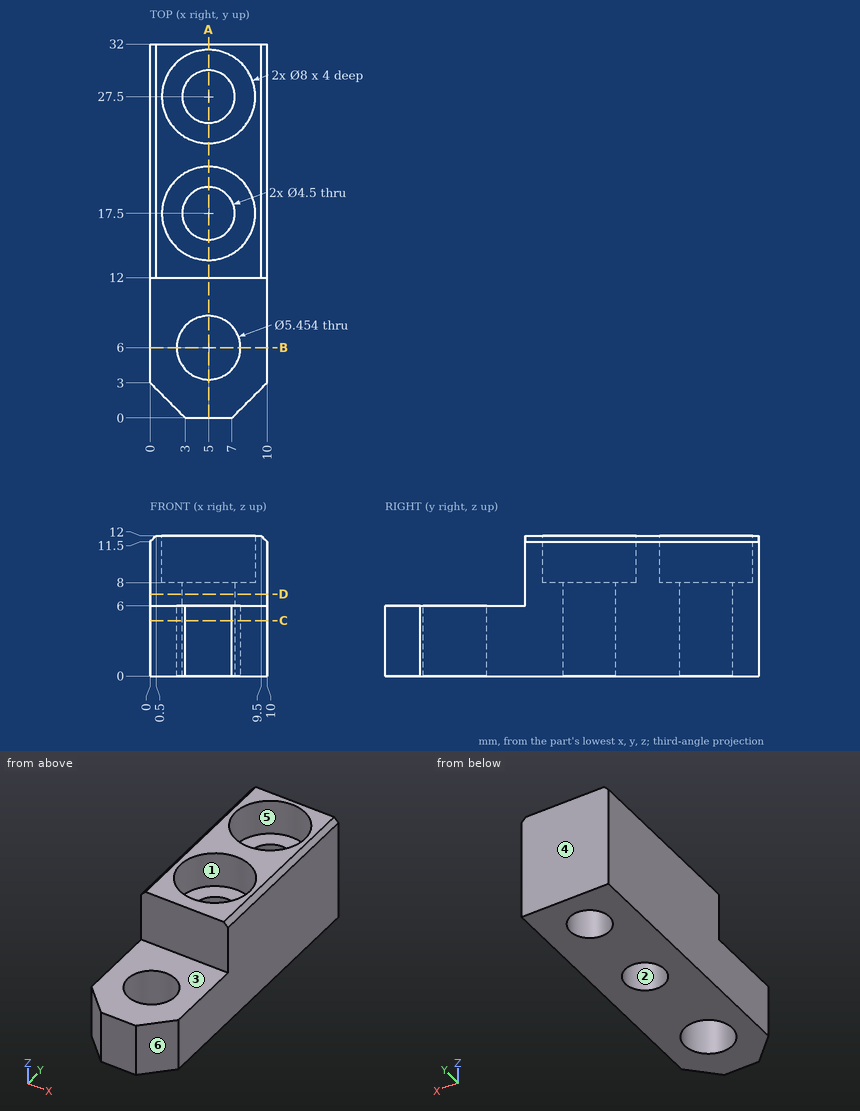
Geometry check sheet. Reference: drawing and pictorial views, mm from the part's lowest x, y, z. A direction names the side the tool comes from. Coordinates: 2 decimals unless noted, no trailing zeros. Write each loop counter-clockwise with the first axis right and the second up, starting at its lowest first coordinate (ties: lowest second). Pieces come first, ordered by that corner, then holes. Notation, with made-up numbers: (-15.75, -28) - (18.25, -28) arc R6 cw to (18.25, -20) - close; hole circle Ø2 at (4.5, 50.5). An arc over 180 degrees is marked (long way). Write item = value, one per line.
Q1. Cross-section at A-A (x = 5). Enter the section's corners in (y, z), plus the area to 3 significant figures.
Answer:
outline = (0, 0) - (3.27, 0) - (3.27, 6) - (0, 6) - close; (8.73, 0) - (15.25, 0) - (15.25, 8) - (13.5, 8) - (13.5, 12) - (12, 12) - (12, 6) - (8.73, 6) - close; (19.75, 0) - (25.25, 0) - (25.25, 8) - (23.5, 8) - (23.5, 12) - (21.5, 12) - (21.5, 8) - (19.75, 8) - close; (29.75, 0) - (32, 0) - (32, 12) - (31.5, 12) - (31.5, 8) - (29.75, 8) - close
area = 143 mm²
Q2. Cross-section at B-B (y = 6). Enter the section's corners in (x, z).
Answer:
outline = (0, 0) - (2.27, 0) - (2.27, 6) - (0, 6) - close; (7.73, 0) - (10, 0) - (10, 6) - (7.73, 6) - close
Q3. Cross-section at D-D (z = 7). Enter the section's corners in (x, y).
Answer:
outline = (0, 12) - (10, 12) - (10, 32) - (0, 32) - close; hole circle Ø4.5 at (5, 17.5); hole circle Ø4.5 at (5, 27.5)
Q4. Mould release check, pull along Y, two halves, no side actions. Record for the marked faces 4, 5 and 6: released by +Y, released by -Y, zero draft, split by the parting line, or undercut.
Answer:
face_4 = released by +Y
face_5 = undercut
face_6 = released by -Y
Q5. Access from +Z, -Z, +X, -X, +Y, -Y to the whole of each face (thin tool, end or side, straight path). Record for the marked faces 1, 2 and 3.
Answer:
face_1 = +Z
face_2 = +Z, -Z
face_3 = +Z, +X, -X, -Y
Q6. Go/stop test with flat-tipped pins: pin 1 Ø4 at (x, y) = (5, 27.5) entering from +Z; pin 2 Ø5 at (x, y) = (5, 27.5) entering from +Z; pin 3 Ø2 at (x, y) = (3.5, 3.5) entering from -Z; pin 4 Ø5 at (x, y) = (4.5, 7.5) entering from +Z. Record where each tip stops, or that it passes through.
Answer:
pin_1 = through
pin_2 = 8
pin_3 = 0
pin_4 = 6
Q7. Cross-section at C-C (z = 4.75). Give the number of separate pieces and of enclosed holes in the cut face, plus the area to 3 significant figures.
Answer:
separate_pieces = 1
enclosed_holes = 3
area = 256 mm²
Q8. Material ranges on L1, parallel to Y at x = 5, z = 10.95; L2, parallel to Y at x = 5, z = 4.5; L3, parallel to Y at x = 3.5, z = 7.5 (1 decimal), recorded low to high. Write a range as from..to.
Answer:
L1 = 12..13.5, 21.5..23.5, 31.5..32
L2 = 0..3.27, 8.73..15.25, 19.75..25.25, 29.75..32
L3 = 12..15.8, 19.2..25.8, 29.2..32
